Geometry: final body of the model. Coordinates: model frame, mm. Give positions to 0.01 mm unless a question says otherwise; leave off trailing zeros. Order: outer loops, then holes, each group sorted by start corner. A loop starts at its lowest first (then second) coordinate and runs counter-clockwise, first axis right, second up. Notation, with made-up numbers: (22, 0.25) -> (68, 0.25) arc R7 cw to (68, 11.25) -> close; hole circle Ø1 at (-19, -4.5). An arc over 180 degrees is marked (long way). Answer in a Markdown table with one row per item. Add a question column.
Q1. Contact query for flat-ended pins moving along their axis: P1, Ø0.6, axis at x = 27, y = -1, coming from the +Z side; P2, Ø3, axis at x = 5.5, y = 5, coming from the +Z side; P3, Ø2, axis at x = 26.5, z = -6.5, coming from the -Y side; P4, Ø8, axis at x = 13, z = 0.5, coming from the +Y side. Output: stop coordinate, or through.
Q2. Line query: line 1 along Z through (x, y) = (-10.5, 19) (3 decimals); line 2 along Y through (x, z) = (-25, -9.5); line 3 along Y through (x, z) = (-31.5, -7). Output: solid intervals per line, ascending. Write a range as from..to.
Q3. Cut plane B-B on y = 14. Return the cut outline in (x, z) (3 decimals), and give its area (3 significant figures).
Q4. Cut plane A-A on x = 14. Return the cut outline in (y, z).
Autodesk Inventor part; units mm, degrees
ref_plane "YZ Plane" through (0, 0, 0) normal (1, 0, 0) x (0, 1, 0)
ref_plane "XZ Plane" through (0, 0, 0) normal (0, 1, 0) x (-1, 0, 0)
ref_plane "XY Plane" through (0, 0, 0) normal (0, 0, 1) x (1, 0, 0)
sketch "Sketch1" plane through (0, 0, 0) normal (0, 1, 0) x (-1, 0, 0)
  line L0 (35.089, 11.43) -> (-35.089, 11.43)
  line L1 (-35.089, 11.43) -> (-35.089, -11.43)
  line L2 (-35.089, -11.43) -> (35.089, -11.43)
  line L3 (35.089, -11.43) -> (35.089, 11.43)
  line L4 (35.089, 11.43) -> (-35.089, -11.43) construction
  line L5 (-35.089, 11.43) -> (35.089, -11.43) construction
  point P0 (0, 0)
  dimension "d0" = 70.178
  dimension "d1" = 22.86
extrude "Extrusion1" add sketch "Sketch1" along normal blind 1.6
fillet "Fillet1" radius 2 4 edges at (-35.089, 0.8, -11.43) (-35.089, 0.8, 11.43) (35.089, 0.8, 11.43) (35.089, 0.8, -11.43)
sketch "Sketch7" plane through (0, 0, 0) normal (0, -1, 0) x (1, 0, 0)
  line L0 (-34.239, 0.97) -> (-27.939, 0.97)
  line L1 (-27.939, 0.97) -> (-27.939, -7.03)
  line L2 (-27.939, -7.03) -> (-34.239, -7.03)
  line L3 (-34.239, -7.03) -> (-34.239, 0.97)
  line L4 (-27.239, 0.97) -> (-20.939, 0.97)
  line L5 (-20.939, 0.97) -> (-20.939, -7.03)
  line L6 (-20.939, -7.03) -> (-27.239, -7.03)
  line L7 (-27.239, -7.03) -> (-27.239, 0.97)
  line L8 (-20.239, 0.97) -> (-13.939, 0.97)
  line L9 (-13.939, 0.97) -> (-13.939, -7.03)
  line L10 (-13.939, -7.03) -> (-20.239, -7.03)
  line L11 (-20.239, -7.03) -> (-20.239, 0.97)
  line L12 (-13.239, 0.97) -> (-6.939, 0.97)
  line L13 (-6.939, 0.97) -> (-6.939, -7.03)
  line L14 (-6.939, -7.03) -> (-13.239, -7.03)
  line L15 (-13.239, -7.03) -> (-13.239, 0.97)
  line L16 (33.089, -11.43) -> (-33.089, -11.43)
  line L17 (-35.089, -9.43) -> (-35.089, 9.43)
  point P0 (0, 0)
  point P1 (-31.089, 0.97)
  point P2 (-24.089, 0.97)
  point P3 (-17.089, 0.97)
  point P4 (-10.089, 0.97)
  point P5 (-34.239, -3.03)
  dimension "d48" = 8
  dimension "d49" = 6.3
  dimension "d50" = 6.3
  dimension "d51" = 6.3
  dimension "d52" = 6.3
  dimension "d53" = 7
  dimension "d54" = 7
  dimension "d55" = 7
  dimension "d56" = 8.4
  dimension "d85" = 4
extrude "Extrusion6" add sketch "Sketch7" along normal blind 2.6
sketch "Sketch8" plane through (0, -2.6, 0) normal (0, -1, 0) x (1, 0, 0)
  circle A0 centre (-31.089, -3.03) radius 1.5
  line L0 (-27.939, 0.97) -> (-34.239, 0.97)
  line L1 (-34.239, 0.97) -> (-34.239, -7.03)
  circle A1 centre (-24.089, -3.03) radius 1.5
  circle A2 centre (-17.089, -3.03) radius 1.5
  circle A3 centre (-10.089, -3.03) radius 1.5
  point P0 (0, 0)
  point P1 (-31.089, 0.97)
  point P2 (-34.239, -3.03)
  dimension "d60" = 3
  dimension "d63" = 7
extrude "Extrusion7" add sketch "Sketch8" along normal blind 1.7
fillet "Fillet2" radius 0.5 4 edges at (-32.589, -2.6, -3.03) (-25.589, -2.6, -3.03) (-18.589, -2.6, -3.03) (-11.589, -2.6, -3.03)
sketch "Sketch9" plane through (0, 0, 0) normal (0, -1, 0) x (1, 0, 0)
  line L0 (25.289, 8.93) -> (29.089, 8.93)
  line L1 (29.089, 8.93) -> (29.089, 5.83)
  line L2 (29.089, 5.83) -> (25.289, 5.83)
  line L3 (25.289, 5.83) -> (25.289, 8.93)
  line L4 (25.289, 0.83) -> (29.089, 0.83)
  line L5 (29.089, 0.83) -> (29.089, 3.93)
  line L6 (29.089, 3.93) -> (25.289, 3.93)
  line L7 (25.289, 3.93) -> (25.289, 0.83)
  line L8 (-33.089, 11.43) -> (33.089, 11.43)
  line L9 (35.089, 9.43) -> (35.089, -9.43)
  point P0 (0, 0)
  dimension "d71" = 3.8
  dimension "d72" = 3.1
  dimension "d73" = 3.1
  dimension "d74" = 1.9
  dimension "d75" = 2.5
  dimension "d76" = 6
extrude "Extrusion8" add sketch "Sketch9" along normal blind 2
sketch "Sketch10" plane through (0, 1.6, 0) normal (0, 1, 0) x (1, 0, 0)
  line L0 (-25.589, -9.505) -> (-10.389, -9.505)
  line L1 (-10.389, -9.505) -> (-10.389, -7.005)
  line L2 (-10.389, -7.005) -> (-25.589, -7.005)
  line L3 (-25.589, -7.005) -> (-25.589, -9.505)
  line L4 (-33.089, -11.43) -> (33.089, -11.43)
  line L5 (-35.089, 9.43) -> (-35.089, -9.43)
  point P0 (0, 0)
  point P1 (-25.589, -8.255)
  dimension "d79" = 3.175
  dimension "d80" = 2.5
  dimension "d81" = 15.2
  dimension "d82" = 9.5
extrude "Extrusion9" add sketch "Sketch10" along normal blind 22
properties part number "Platine"
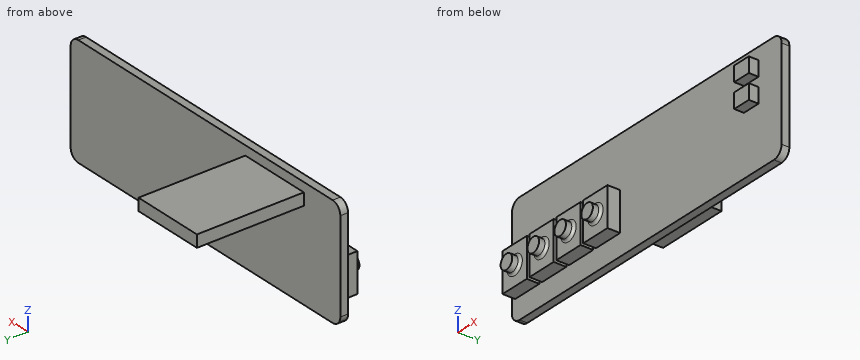
Completed:
| question | item | result |
|---|---|---|
| 1 | P1 | stops at z = 8.93 |
| 1 | P2 | passes through |
| 1 | P3 | stops at y = 0 |
| 1 | P4 | stops at y = 1.6 |
| 2 | line 1 | z = 7.005..9.505 |
| 2 | line 2 | y = 0..1.6 |
| 2 | line 3 | y = -2.6..1.6 |
| 3 | outline | (-25.589, 7.005) -> (-10.389, 7.005) -> (-10.389, 9.505) -> (-25.589, 9.505) -> close |
| 3 | area | 38.0 mm² |
| 4 | outline | (0, -11.43) -> (1.6, -11.43) -> (1.6, 11.43) -> (0, 11.43) -> close |
